The model under review builds one solid part; all positions refer to its coordinate system, in mm. Face numbers are marked on the shaded views. A direction names the side the tool comes from. Coordinates: 2 decimals unless noted, no trailing zeros. Order: outer loops, then holes, each group sorted by start corner. A loop starts at its lowest first (then second) coordinate and runs counter-clockwise, first axis right, second up. Notation, with made-up numbers: (12.25, 73) -> (49.25, 73) arc R18 cw to (49.25, 106) -> close; hole circle Ø3 at (10.5, 2). An arc over 180 degrees is marked (long way). Use one line per item in the form item = value.
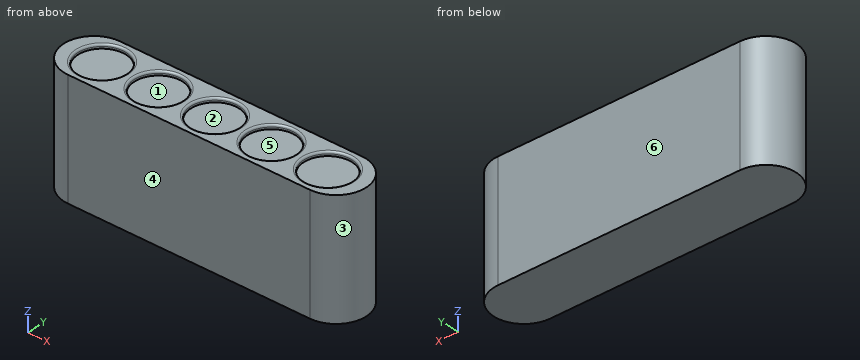
from build123d import *

# Parameters (mm, degrees)
BOSS_EXTRUDE1_DEPTH = 58
SKETCH2_R           = 12
CUT_EXTRUDE1_DEPTH  = 2
FILLET1_R           = 1


with BuildPart() as part:
    # Sketch1 → Boss-Extrude1 (new body)
    with BuildSketch(Plane.XY):
        with BuildLine():
            Line((120, 15), (0, 15))
            ThreePointArc((0, 15), (-15, 0), (0, -15))
            Line((0, -15), (120, -15))
            ThreePointArc((120, -15), (135, 0), (120, 15))
        make_face()
    extrude(amount=BOSS_EXTRUDE1_DEPTH)

    # Sketch2 → Cut-Extrude1 (cut)
    with BuildSketch(Plane.XY.offset(58)):
        with Locations((60, 0)):
            Circle(SKETCH2_R)
        with Locations((88, 0)):
            Circle(SKETCH2_R)
        with Locations((116, 0)):
            Circle(SKETCH2_R)
        with Locations((32, 0)):
            Circle(SKETCH2_R)
        with Locations((4, 0)):
            Circle(SKETCH2_R)
    extrude(amount=-CUT_EXTRUDE1_DEPTH, mode=Mode.SUBTRACT)

    # Fillet1
    fillet1_edges = [part.edges().sort_by_distance(p)[0] for p in [
        (-8, 0, 58),
        (20, 0, 58),
        (104, 0, 58),
        (76, 0, 58),
        (48, 0, 58),
    ]]
    fillet(fillet1_edges, radius=FILLET1_R)


solid = part.part
Item 1: Clearance check with flat-ended pins moving along their axes: pin 1 (7 mm diameter, centred on x = 0, y = 0.5, fed in from +Z); pin 2 (1 mm diameter, centred on y = 8.5, z = 28, fed in from -X). State where each tip first meets the part, or that it passes through.
Results found:
pin_1 = 56
pin_2 = -12.69
Item 2: We need section C-C (z = 36). Write out the cut boundary in (x, y).
Results found:
outline = (0, -15) -> (120, -15) arc R15 ccw to (120, 15) -> (0, 15) arc R15 ccw to start
Item 3: We need section A-A (x = 32). Write out the cut boundary in (y, z), plus the area to 3 significant figures.
Results found:
outline = (-15, 0) -> (15, 0) -> (15, 58) -> (13, 58) arc R1 ccw to (12, 57) -> (12, 56) -> (-12, 56) -> (-12, 57) arc R1 ccw to (-13, 58) -> (-15, 58) -> close
area = 1,690 mm²
Item 4: Draft analysis for pull direction X (two halves, no side actions). For the marked faces 1, 2, 3 and 4, state which applies: released by +X, released by -X, zero draft, split by the parting line, or undercut.
Results found:
face_1 = undercut
face_2 = undercut
face_3 = released by +X
face_4 = zero draft
Item 5: To check wall thickness, follow L1, parallel to Y at x = 60, z = 56.6; L2, parallel to Z at x = 52, y = 2; L3, parallel to X at y = 0.5, z = 4. State the ranges of each line that lie inside material, in increasing order. Write a range as from..to.
Results found:
L1 = -15..-12, 12..15
L2 = 0..56
L3 = -14.99..134.99
Item 6: Tool access review of the marked faces 5 and 6: name each direction out of +Z, -Z, +X, -X, +Y, -Y from which nothing blocks a thin tool from reaching the whole face with its end or side.
Results found:
face_5 = +Z
face_6 = +Z, -Z, +X, -X, +Y
